Source: CAD feature listing. Evaluate the final solid. Frame: model axes, mm. A direction names the side the tool comes from. Round coordinates to 2 decimals unless told otherwise and drop trailing zeros. Order: outer loops, then holes, each group sorted by start corner. A loop starts at its lowest first (then second) coordinate and runs counter-clockwise, first axis right, second up. Notation, with made-up numbers: (75, 68) - (124, 68) arc R23 ccw to (124, 97) - close; hole circle Ø10 at (2.25, 19). An arc over 180 degrees is marked (long way). Put each result on its own line as item: value. Start each with the question number.
1) Contact query for flat-ended pins moving along their axis: P1, Ø10, axis at y = -7.5, z = 43.5, coming from the +X side; P2, Ø2, axis at x = -5.5, y = 6.5, coming from the -Z side; P3, Ø3, axis at x = -1.5, z = 54.5, coming from the -Y side; P4, Ø10, axis at x = -2, y = 2.5, coming from the +Z side. Output: stop coordinate, or through.
2) Section B-B on z = 52. Output: boundary loops of the cut face in (x, y), then the cut area to 3 significant figures.
3) Access query for faces 5 (the face through (-1.3, -1.1, 54.5)), 6 (the face through (0, 0, -3.5)). Directions: +Z, -Z, +X, -X, +Y, -Y. A direction counts if a zero-diameter tool reaches every point of the face in a straight line with its end or side. Return the directions, or none.
4) Line query: probe 1 along Y at (x, z) = (0, 46); probe 2 along Z at (x, y) = (11.5, -0.5); probe 3 along X at (y, z) = (-0.5, 34.5). Output: solid intervals per line, ascending. Write a range as [from, to].
5) Section A-A on z = 41. Output: boundary loops of the cut face in (x, y), then the cut area to 3 significant figures.
6) Mould query, pull axis Y, two halves, no side actions, for faces 1 (the face through (8, 0, 0)), 2 (the face through (0, -12, 45)), 3 (the face through (0, 13, 45)), 4 (the face through (5.158, 3.955, -0.986)). Classes: +Y half, -Y half, draft (parallel to the pull), parting line (faces both ways), or undercut.
Autodesk Inventor part; units mm, degrees
ref_plane "YZ Plane" through (0, 0, 0) normal (1, 0, 0) x (0, 1, 0)
ref_plane "XZ Plane" through (0, 0, 0) normal (0, 1, 0) x (-1, 0, 0)
ref_plane "XY Plane" through (0, 0, 0) normal (0, 0, 1) x (1, 0, 0)
sketch "Эскиз1" plane through (0, 0, 0) normal (0, 0, 1) x (1, 0, 0)
  circle A0 centre (0, 0) radius 17.85
  dimension "d37" = 35.7
extrude "Выдавливание1" add sketch "Эскиз1" along normal blind 50
sketch "Sketch7" plane through (0, 0, 50) normal (0, 0, 1) x (1, 0, 0)
  circle A0 centre (0, 0) radius 6.5
  dimension "d40" = 13
extrude "Extrusion7" add sketch "Sketch7" along normal blind 4.5
sketch "Sketch8" plane through (0, 0, 54.5) normal (0, 0, 1) x (1, 0, 0)
  circle A0 centre (0, 0) radius 1.5
  dimension "d43" = 3
extrude "Extrusion8" add sketch "Sketch8" along normal blind 9
sketch "Sketch10" plane through (0, 0, 50) normal (0, 0, 1) x (1, 0, 0)
  circle A0 centre (0, 12.5) radius 1.5
  circle A1 centre (0, -12.5) radius 1.5
  point P0 (0, 0)
  dimension "d53" = 3
  dimension "d54" = 3
  dimension "d58" = 12.5
  dimension "d59" = 12.5
extrude "Extrusion9" cut sketch "Sketch10" against normal blind 5
thread "Thread1"
thread "Thread2"
sketch "Sketch12" plane through (0, 0, 0) normal (0, 0, -1) x (-1, 0, 0)
  circle A0 centre (0, 0) radius 6.5
  dimension "d67" = 13
extrude "Extrusion10" add sketch "Sketch12" along normal blind 3
sketch "Sketch13" plane through (0, 0, -3) normal (0, 0, -1) x (-1, 0, 0)
  circle A0 centre (0, 0) radius 1.25
  dimension "d70" = 2.5
extrude "Extrusion11" add sketch "Sketch13" along normal blind 0.5
fillet "Fillet3" radius 1 1 edges at (6.5, 0, -3)
fillet "Fillet4" radius 0.3 1 edges at (1.25, 0, -3.5)
fillet "Fillet5" radius 1 1 edges at (-6.5, 0, 54.5)
sketch "Sketch14" plane through (0, 0, 0) normal (0, 0, -1) x (-1, 0, 0)
  line L0 (14.85, -1.5) -> (14.35, -1.5)
  line L1 (14.35, -1.5) -> (14.35, 1.5)
  line L2 (14.35, 1.5) -> (14.85, 1.5)
  line L3 (14.85, 1.5) -> (14.85, -1.5)
  line L4 (-14.35, -1.5) -> (-14.85, -1.5)
  line L5 (-14.85, -1.5) -> (-14.85, 1.5)
  line L6 (-14.85, 1.5) -> (-14.35, 1.5)
  line L7 (-14.35, 1.5) -> (-14.35, -1.5)
  line L8 (0, 0) -> (18.9187, 0)
  circle A0 centre (0, 0) radius 1.5
  line L9 (0, 0) -> (-19.0249, 0)
  dimension "d76" = 0.5
  dimension "d77" = 0.5
  dimension "d78" = 28.7
  dimension "d79" = 14.35
  dimension "d80" = 3
extrude "Extrusion12" add sketch "Sketch14" along normal blind 6 contours L0 L1 L8 L3 | L8 L1 L2 L3 | L4 L5 L9 L7 | L9 L5 L6 L7
fillet "Fillet6" radius 1.5 4 edges at (-14.6, -1.5, -6) (-14.6, 1.5, -6) (14.6, -1.5, -6) (14.6, 1.5, -6)
sketch "Sketch15" plane through (-14.85, -1.5, 0) normal (-1, 0, 0) x (0, 0, 1)
  line L0 (-1, 0.5) -> (-4.5, 0.5)
  line L1 (-4.5, 2.5) -> (-1, 2.5)
  line L2 (-1, 2.5) -> (-1, 0.5)
  line L3 (0, 0) -> (-4.5, 0)
  line L4 (0, 3) -> (-4.5, 3)
  line L5 (0, -16.35) -> (0, 19.35)
  arc A0 (-4.5, 2.5) -> (-4.5, 0.5) centre (-4.5, 1.5) ccw
  point P0 (0, 1.5)
  dimension "d84" = 0.5
  dimension "d85" = 0.5
  dimension "d86" = 1
  dimension "d87" = 3.5
  dimension "d88" = 3.5
  dimension "d89" = 1
extrude "Extrusion13" cut sketch "Sketch15" against normal blind 1
sketch "Sketch16" plane through (14.85, -1.5, 0) normal (1, 0, 0) x (0, 0, -1)
  line L0 (1, 2.5) -> (1, 0.5)
  line L1 (1, 2.5) -> (4.5, 2.5)
  line L2 (1, 0.5) -> (4.5, 0.5)
  line L3 (4.5, 2.5) -> (1, 2.5)
  line L4 (1, 2.5) -> (1, 0.5)
  arc A0 (4.5, 0.5) -> (4.5, 2.5) centre (4.5, 1.5) ccw
  arc A1 (4.5, 0.5) -> (4.5, 2.5) centre (4.5, 1.5) ccw
  point P0 (0, 1.5)
  dimension "d92" = 1
extrude "Extrusion14" cut sketch "Sketch16" against normal blind 1
fillet "Fillet7" radius 1 1 edges at (-17.85, 0, 50)
properties part number "R370-25120" material "Stainless Steel, 440C"
Answer sheet:
1. P1: x = 17.67
1. P2: z = 0
1. P3: y = -6.49
1. P4: z = 63.5
2. outline: circle Ø13 at (0, 0)
2. area: 133 mm^2
3. face 5: +Z
3. face 6: -Z, +X, -X, +Y, -Y
4. probe 1: [-17.85, -14], [-11, 11], [14, 17.85]
4. probe 2: [0, 50]
4. probe 3: [-17.84, 17.84]
5. outline: circle Ø35.7 at (0, 0)
5. area: 1,000 mm^2
6. face 1: draft
6. face 2: undercut
6. face 3: undercut
6. face 4: parting line
